Read the model definition and answer for the solid it produces. Units are mm, in the model's axes. Face numbers are marked on the shaded views. A direction names the side the tool comes from. Give positions to 0.01 mm unless a question says otherwise; leave off trailing zeros. Loops run counter-clockwise (first coordinate to the right, second up) from the corner with the lowest first, then second, coordinate; pieces in that order, holes last.
(1) Find section D-D, the plane z = -5. Write down the section's boundary in (x, y).
(2) Find section C-C, the plane y = -1. Write down the section's boundary in (x, z).
(3) Find section A-A, the plane x = 5. State how many separate pieces and enclosed holes the cut face has, then the cut area to 3 significant figures.
(4) Which of the six approach directions +Z, -Z, +X, -X, +Y, -Y give full straight-line access (tool end or side, diameter ignored) to the marked faces 1, 2, 3, 4 and 5?
(5) Straight lines are drawn through the part: probe 1 along Y at (x, z) = (2, 0); probe 2 along Z at (x, y) = (0, -3); probe 3 along Y at (x, z) = (1.5, -3.5). For each, find the intervals that lie inside material, in ascending order.
(6) Each of these flat-tipped pins is pushed along its axis until it touches: P1, Ø5, axis at x = 2, y = -2, coming from the +Z side; P2, Ø6, axis at y = 9, z = -3, coming from the +X side; P3, Ø1.6, axis at x = 4.5, z = 1, coming from the +Y side. Where does it stop, or does it pass through?
(7) Find section B-B, the plane y = 14.5. Write down the section's boundary in (x, z).
(8) Determine the mould class of the marked faces 6, 7 and 8 for opening direction Z: pulls with the +Z half, pulls with the -Z half, needs draft (parallel to the pull), parting line crosses it, or undercut.
Autodesk Inventor part; units mm, degrees
ref_plane "YZ Plane" through (0, 0, 0) normal (1, 0, 0) x (0, 1, 0)
ref_plane "XZ Plane" through (0, 0, 0) normal (0, 1, 0) x (-1, 0, 0)
ref_plane "XY Plane" through (0, 0, 0) normal (0, 0, 1) x (1, 0, 0)
sketch "Sketch1" plane through (0, 0, 0) normal (0, 0, 1) x (1, 0, 0)
  line L0 (0, 18.75) -> (6.2, 18.75)
  line L1 (6.2, -18.75) -> (0, -18.75)
  line L2 (0, -18.75) -> (0, 18.75)
  line L3 (0, 8.7) -> (8, 8.7)
  line L4 (8, 8.7) -> (8, -8.7)
  line L5 (8, -8.7) -> (0, -8.7)
  line L6 (0, -8.7) -> (0, 8.7)
  line L7 (6.2, 11.4) -> (26.2, 11.4)
  line L8 (26.2, 11.4) -> (26.2, -11.4)
  line L9 (26.2, -11.4) -> (6.2, -11.4)
  line L10 (6.2, 18.75) -> (6.2, 11.4)
  line L11 (6.2, -11.4) -> (6.2, -18.75)
  line L12 (6.2, 11.4) -> (6.2, -11.4) construction
  line L13 (0, 0) -> (26.2, 0) construction
  point P0 (6.2, 0)
  dimension "d0" = 37.5
  dimension "d1" = 6.2
  dimension "d2" = 17.4
  dimension "d3" = 8
  dimension "d4" = 20
  dimension "d5" = 22.8
extrude "Extrusion1" add sketch "Sketch1" along normal mid plane 12 contours L0 L10 L7 L8 L9 L11 L1 L2 L5 L4 L3
sketch "Sketch2" plane through (0, 0, 0) normal (1, 0, 0) x (0, 1, 0)
  line L0 (14, 0) -> (-14, 0) construction
  circle A0 centre (14, 0) radius 1.5
  circle A1 centre (-14, 0) radius 1.5
  point P0 (0, 0)
  point P1 (0, 0)
  dimension "d8" = 28
  dimension "d9" = 3
extrude "Extrusion2" cut sketch "Sketch2" along normal through all
sketch "Sketch3" plane through (8, -8.7, -6) normal (-1, 0, 0) x (0, 0, 1)
  line L0 (9.75, 16.2) -> (2.25, 16.2)
  line L1 (2.25, 16.2) -> (2.25, 1.2)
  line L2 (2.25, 1.2) -> (9.75, 1.2)
  line L3 (9.75, 1.2) -> (9.75, 16.2)
  line L4 (9.75, 16.2) -> (2.25, 1.2) construction
  line L5 (2.25, 16.2) -> (9.75, 1.2) construction
  line L6 (2.75, 15.7) -> (9.25, 15.7)
  line L7 (9.25, 15.7) -> (9.25, 1.7)
  line L8 (9.25, 1.7) -> (2.75, 1.7)
  line L9 (2.75, 1.7) -> (2.75, 15.7)
  line L10 (2.75, 15.7) -> (9.25, 1.7) construction
  line L11 (9.25, 15.7) -> (2.75, 1.7) construction
  line L12 (8.25, 15.2) -> (6.25, 15.2)
  line L13 (6.25, 15.2) -> (6.25, 2.2)
  line L14 (6.25, 2.2) -> (8.25, 2.2)
  line L15 (8.25, 2.2) -> (8.25, 15.2)
  line L16 (8.25, 15.2) -> (6.25, 2.2) construction
  line L17 (6.25, 15.2) -> (8.25, 2.2) construction
  line L18 (7.25, 8.7) -> (6, 8.7) construction
  dimension "d12" = 7.5
  dimension "d13" = 15
  dimension "d14" = 0.5
  dimension "d15" = 0.5
  dimension "d16" = 2
  dimension "d17" = 1
  dimension "d18" = 0.5
extrude "Extrusion3" add sketch "Sketch3" along normal blind 9.5
fillet "Fillet1" radius 6 6 edges at (3.1, 18.75, 6) (3.1, 18.75, -6) (3.1, -18.75, 6) (3.1, -18.75, -6) (26.2, -11.4, 0) (26.2, 11.4, 0)
properties part number "panel-usb" material "Rubber"
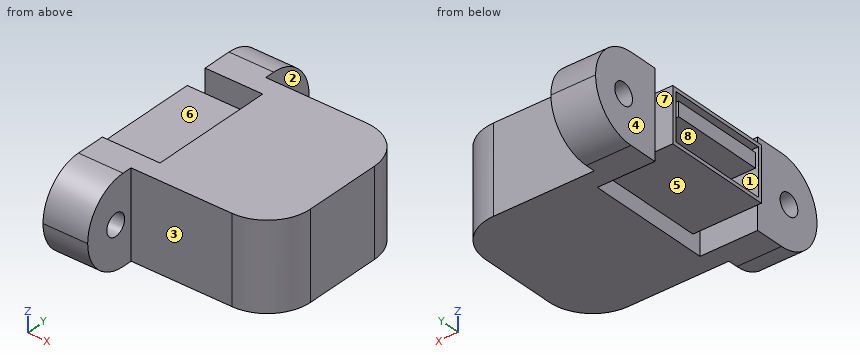
Entries:
1. outline: (0, -16.07) - (6.2, -16.07) - (6.2, -11.4) - (20.2, -11.4) arc R6 ccw to (26.2, -5.4) - (26.2, 5.4) arc R6 ccw to (20.2, 11.4) - (6.2, 11.4) - (6.2, 16.07) - (0, 16.07) - (0, 8.7) - (8, 8.7) - (8, -8.7) - (0, -8.7) - close
2. outline: (-1.5, -3.75) - (8, -3.75) - (8, -6) - (26.2, -6) - (26.2, 6) - (8, 6) - (8, 3.75) - (-1.5, 3.75) - (-1.5, 3.25) - (8, 3.25) - (8, 2.25) - (-1.5, 2.25) - (-1.5, 0.25) - (8, 0.25) - (8, -3.25) - (-1.5, -3.25) - close
3. separate pieces: 4
3. enclosed holes: 3
3. area: 244 mm2
4. face 1: -X
4. face 2: +Z, -Z, +X, +Y
4. face 3: +Z, -Z, +X, -Y
4. face 4: +Z, -Z, -X, +Y
4. face 5: -Z, -X
5. probe 1: y = -18.75 to -15.5, -12.5 to -8.7, -7.5 to -7, 7 to 7.5, 8.7 to 12.5, 15.5 to 18.75
5. probe 2: z = -3.75 to -3.25, 0.25 to 2.25, 3.25 to 3.75
5. probe 3: y = -17.62 to -8.7, -7.5 to 7.5, 8.7 to 17.62
6. P1: stops at z = 3.75
6. P2: stops at x = 26.17
6. P3: stops at y = 18.75
7. outline: (0, -5.74) - (6.2, -5.74) - (6.2, -1.41) - (0, -1.41) - close; (0, 1.41) - (6.2, 1.41) - (6.2, 5.74) - (0, 5.74) - close
8. face 6: pulls with the +Z half
8. face 7: needs draft
8. face 8: undercut
